CAD build for the part. Positions are in the model's coordinates, mm. Round coordinates to 2 decimals unless told otherwise and drop trailing zeros. Loops run counter-clockwise (first coordinate to the right, second up) from the corner with the lowest first, then second, coordinate; pieces in that order, holes last. Notation, with made-up numbers: M 68,-36 L 90,-36 A28 ccw 90,1 Z; hole C 57,-37 d4. An arc over 180 degrees is marked long. Put each result on its own line as item: value. Start each with the question number.
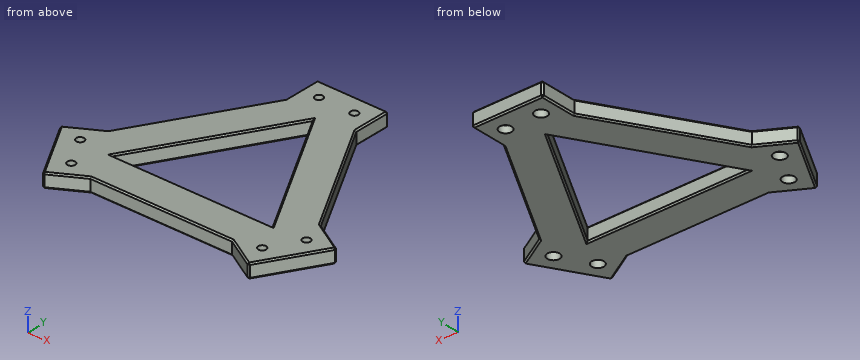
from build123d import *

# Parameters (mm, degrees)
F1_DEPTH       = 20
F2_SIZE        = 40
F3_W           = 100
F3_H           = 51.9615242271
F4_DEPTH       = 20
F5_SIZE        = 2
F7_D           = 11
F7_CBORE_D     = 17.25
F7_CBORE_DEPTH = 10


with BuildPart() as f1:
    # F0 (on Top) → F1 (new body)
    with BuildSketch(Plane.XY):
        Polygon((0, 230.9401076759), (-200, -115.4700538379), (200, -115.4700538379), align=None)
        Polygon((-113.3974596216, -65.4700538379), (0, 130.9401076759), (113.3974596216, -65.4700538379), align=None, mode=Mode.SUBTRACT)
    extrude(amount=-F1_DEPTH)

    # F2
    f2_edges = [f1.edges().sort_by_distance(p)[0] for p in [
        (-200, -115.470054, -10),
        (200, -115.470054, -10),
        (0, 230.940108, -10),
    ]]
    chamfer(f2_edges, length=F2_SIZE)

    # F3 (on face) → F4 (join, through all)
    with BuildSketch(Plane.XY):
        with Locations((0, 170.3183294109)):
            Rectangle(F3_W, F3_H)
        Polygon((-145, -141.4508159515), (-100, -115.4700538379), (-150, -28.8675134595), (-195, -54.848275573), align=None)
        Polygon((195, -54.848275573), (150, -28.8675134595), (100, -115.4700538379), (145, -141.4508159515), align=None)
    extrude(amount=-F4_DEPTH)

    # F5
    f5_edges = [f1.edges().sort_by_distance(p)[0] for p in [
        (-50, 170.318329, -20),
        (-100, 57.735027, -20),
        (-172.5, -41.857895, -20),
        (-170, -98.149546, -20),
        (-122.5, -128.460435, -20),
        (0, -115.470054, -20),
        (122.5, -128.460435, -20),
        (170, -98.149546, -20),
        (172.5, -41.857895, -20),
        (100, 57.735027, -20),
        (50, 170.318329, -20),
        (0, 196.299092, -20),
        (-56.69873, 32.735027, -20),
        (56.69873, 32.735027, -20),
        (0, -65.470054, -20),
        (-50, 170.318329, 0),
        (-100, 57.735027, 0),
        (-172.5, -41.857895, 0),
        (-170, -98.149546, 0),
        (-122.5, -128.460435, 0),
        (0, -115.470054, 0),
        (122.5, -128.460435, 0),
        (170, -98.149546, 0),
        (172.5, -41.857895, 0),
        (100, 57.735027, 0),
        (50, 170.318329, 0),
        (0, 196.299092, 0),
        (-56.69873, 32.735027, 0),
        (56.69873, 32.735027, 0),
        (0, -65.470054, 0),
        (-145, -141.450816, -10),
        (-195, -54.848276, -10),
        (50, 196.299092, -10),
        (-50, 196.299092, -10),
        (145, -141.450816, -10),
        (195, -54.848276, -10),
    ]]
    chamfer(f5_edges, length=F5_SIZE)

    # F7 (through all)
    with Locations(Plane(origin=(0, 0, -20), x_dir=(1, 0, 0), z_dir=(0, 0, -1))):
        with Locations((159.7243186434, 63.3493649054), (134.7243186434, 106.6506350946), (-25, -170), (25, -170), (-134.7243186434, 106.6506350946), (-159.7243186434, 63.3493649054)):
            CounterBoreHole(F7_D / 2, F7_CBORE_D / 2, F7_CBORE_DEPTH)


solid = f1.part
(1) Drill centre lines: line 1 along X through (y, z) = (170, -6.25); line 2 along Y through (x, z) = (-25, -7.5); line 3 along X through (y, z) = (-65, -10.5). Where is each one in solid material? Low to high.
(2) Cut at D-D on y = -44.5. List the corners of the cut face in (x, z), and give its area (3 significant figures).
(3) Cut at A-A on y = 170. List the corners of the cut face in (x, z) (3 decimals).
(4) Flat gauge pins, fed straight in: pin 1 Ø9 at (x, y) = (-159.72, -63.35) entering from -Z; pin 2 Ø8 at (x, z) = (-21, -11) entering from -Y; pin 3 Ø12 at (y, z) = (-90.5, -14.5) entering from -X; pin 4 Ø2 at (y, z) = (50.5, -12) entering from +X. Where does each tip first touch, or does it go through?
(5) Cut at C-C on z = -13.5. List the corners of the cut face in (x, y) (3 decimals), and give its area (3 significant figures).
(6) Cut at B-B on x = -25. List the corners of the cut face in (y, z) (3 decimals), and give its area (3 significant figures).
Taken from the geometry:
1. line 1: -50 to -30.5, -19.5 to 19.5, 30.5 to 50
1. line 2: -115.47 to -65.47, 87.64 to 164.5, 175.5 to 196.3
1. line 3: -189.14 to -168.19, -151.26 to -113.13, 113.13 to 151.26, 168.19 to 189.14
2. outline: M -177.08,-18 L -173.08,-20 L -103.6,-20 L -101.29,-18 L -101.29,-2 L -103.6,0 L -173.08,0 L -177.08,-2 Z; M 101.29,-18 L 103.6,-20 L 173.08,-20 L 177.08,-18 L 177.08,-2 L 173.08,0 L 103.6,0 L 101.29,-2 Z
2. area: 3,010 mm2
3. outline: M -50,-18 L -48,-20 L -33.625,-20 L -33.625,-10 L -30.5,-10 L -30.5,0 L -48,0 L -50,-2 Z; M -19.5,-10 L -16.375,-10 L -16.375,-20 L 16.375,-20 L 16.375,-10 L 19.5,-10 L 19.5,0 L -19.5,0 Z; M 30.5,-10 L 33.625,-10 L 33.625,-20 L 48,-20 L 50,-18 L 50,-2 L 48,0 L 30.5,0 Z
4. pin 1: through
4. pin 2: y = -115.47
4. pin 3: x = -177.88
4. pin 4: x = 104.75
5. outline: M -194,-56.58 L -146,-139.719 L -143.268,-140.451 L -100,-115.47 L 100,-115.47 L 143.268,-140.451 L 146,-139.719 L 194,-56.58 L 193.268,-53.848 L 150,-28.868 L 50,144.338 L 50,194.299 L 48,196.299 L -48,196.299 L -50,194.299 L -50,144.338 L -150,-28.868 L -193.268,-53.848 Z; hole C -159.724,-63.349 d17.25; hole C -134.724,-106.651 d17.25; hole M -113.397,-65.47 L 113.397,-65.47 L 0,130.94 Z; hole C -25,170 d17.25; hole C 25,170 d17.25; hole C 134.724,-106.651 d17.25; hole C 159.724,-63.349 d17.25
5. area: 48,200 mm2
6. outline: M -115.47,-18 L -113.47,-20 L -67.47,-20 L -65.47,-18 L -65.47,-2 L -67.47,0 L -113.47,0 L -115.47,-2 Z; M 87.639,-18 L 91.639,-20 L 161.375,-20 L 161.375,-10 L 164.5,-10 L 164.5,0 L 91.639,0 L 87.639,-2 Z; M 175.5,-10 L 178.625,-10 L 178.625,-20 L 194.299,-20 L 196.299,-18 L 196.299,-2 L 194.299,0 L 175.5,0 Z
6. area: 2,870 mm2
